Source: three-view drawing plus pictorial views. Frame: mm from the lowest corner of the part. A direction names the side the tool comes from. Give positions to 0.01 mm unless a question says otherwise; leave off trailing zeros. Loops run counter-clockwise (first coordinate to the right, second up) from the corner with the lowest first, then second, coordinate; pieces in that order, holes last. Notation, with made-up numbers: (-40, 10.5) - (-32, 10.5) arc R23 cw to (-32, 29.5) - close; hole circle Ø9 at (62, 60.25). An arc over 180 degrees is marked (long way). Answer in a Markdown table with one row per item.
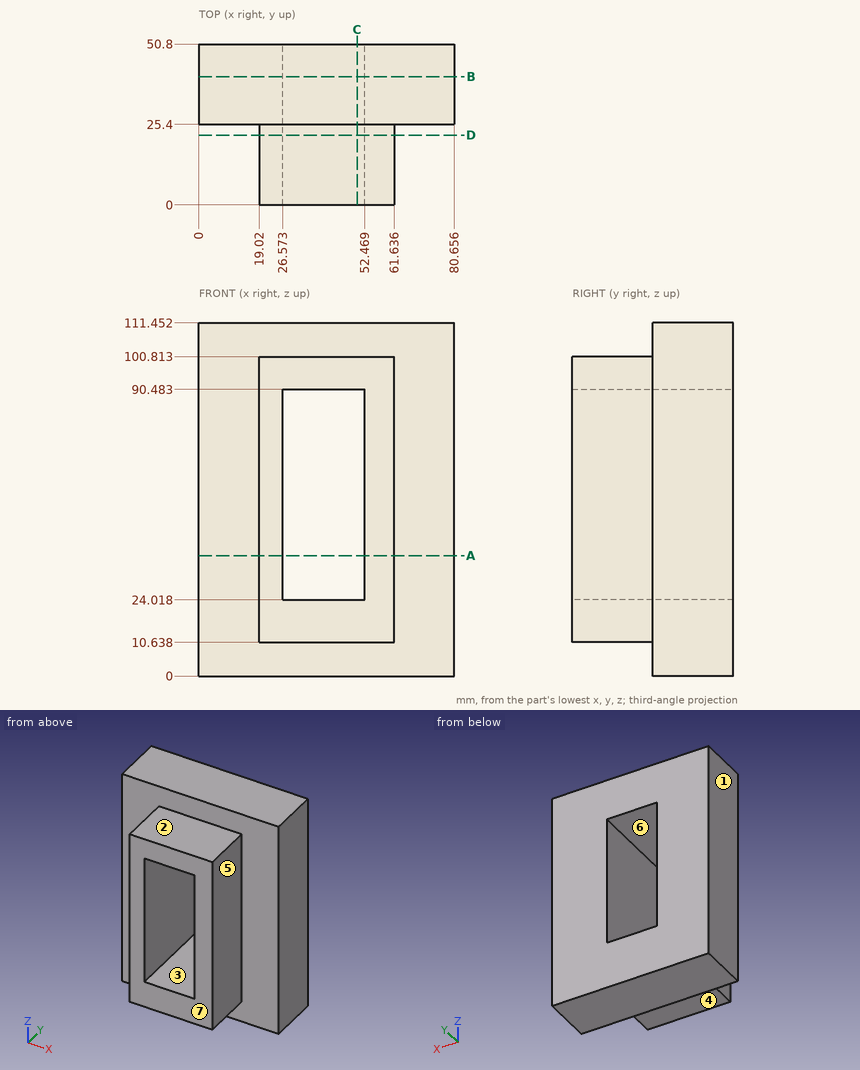
Q1. Cut plane B-B (y = 40.5). Output: boundary loops of the cut face in (x, z) (1 decimal).
Check values:
| item | result |
|---|---|
| outline | (0, 0) - (80.7, 0) - (80.7, 111.5) - (0, 111.5) - close; hole (26.6, 24) - (52.5, 24) - (52.5, 90.5) - (26.6, 90.5) - close |
Q2. Cut plane C-C (x = 50). Output: boundary loops of the cut face in (y, z).
Check values:
| item | result |
|---|---|
| outline | (0, 10.64) - (25.4, 10.64) - (25.4, 0) - (50.8, 0) - (50.8, 24.02) - (0, 24.02) - close; (0, 90.48) - (50.8, 90.48) - (50.8, 111.45) - (25.4, 111.45) - (25.4, 100.81) - (0, 100.81) - close |
Q3. Cut plane D-D (y = 22). Output: boundary loops of the cut face in (x, z) (1 decimal).
Check values:
| item | result |
|---|---|
| outline | (19, 10.6) - (61.6, 10.6) - (61.6, 100.8) - (19, 100.8) - close; hole (26.6, 24) - (52.5, 24) - (52.5, 90.5) - (26.6, 90.5) - close |
Q4. Cut plane A-A (z = 38). Output: boundary loops of the cut face in (x, y) (1 decimal), and give its area (3 significant figures).
Check values:
| item | result |
|---|---|
| outline | (0, 25.4) - (19, 25.4) - (19, 0) - (26.6, 0) - (26.6, 50.8) - (0, 50.8) - close; (52.5, 0) - (61.6, 0) - (61.6, 25.4) - (80.7, 25.4) - (80.7, 50.8) - (52.5, 50.8) - close |
| area | 1,820 mm² |
Q5. Reachability of the marked faces 1, 2, 3 and 4 from +Z, -Z, +X, -X, +Y, -Y: full face, straight path, thin tool, end or side. Return the list, or none.
Check values:
| item | result |
|---|---|
| face 1 | +Z, -Z, -X, +Y, -Y |
| face 2 | +Z, +X, -X, -Y |
| face 3 | +Y, -Y |
| face 4 | -Z, +X, -X, -Y |
Q6. Material intervals for line 1 along X through (y, z) = (18.5, 28) (1 decimal); line 2 along X through (y, z) = (45.5, 72) (1 decimal); line 3 along Z through (x, y) = (50, 13), sorted ascending.
Check values:
| item | result |
|---|---|
| line 1 | 19 to 26.6, 52.5 to 61.6 |
| line 2 | 0 to 26.6, 52.5 to 80.7 |
| line 3 | 10.64 to 24.02, 90.48 to 100.81 |
Q7. Draft query along X for the marked faces 5, 6 and 7. Return one class per face: pulls with the +X half, pulls with the -X half, needs draft (parallel to the pull), parting line crosses it, or undercut.
Check values:
| item | result |
|---|---|
| face 5 | pulls with the +X half |
| face 6 | undercut |
| face 7 | needs draft |
Q8. First-contact query: pin 1 (4 mm diameter, centred on x = 23.5, y = 11, fed in from +Z); pin 2 (20.5 mm diameter, centred on y = 8, z = 64.5, fed in from -X); pin 3 (4 mm diameter, centred on x = 12, z = 39, fed in from -Y). Flat tips, straight axial feed; report the tip coordinate or a pass-through.
Check values:
| item | result |
|---|---|
| pin 1 | z = 100.81 |
| pin 2 | x = 19.02 |
| pin 3 | y = 25.4 |
